Design review of the part built by this model. Coordinates are the model's own, in mm. Round coordinates to 2 decimals unless told otherwise and drop trailing zeros. Loops run counter-clockwise (first coordinate to the right, second up) from the corner with the lowest first, then second, coordinate; pieces in that order, holes last. Notation, with made-up numbers: (-15.5, 30) - (23.5, 30) arc R29 cw to (23.5, 63) - close; hole circle Ø4 at (-5.75, 14). An arc over 180 degrees is marked (long way). Return JSON: item names as keys, results as strings. Group by question number.
(1) We need section A-A, the plane x = -257.5. Write out the cut boundary in (y, z).
(2) Wall thickness on L1, parallel to Z at x = -230, y = 3.05; L2, parallel to Z at x = -247, y = 1.85; L3, parallel to X at y = 1, z = -209: over which ranges is each line inside the solid? List them lowest first. Write a range as [from, to].
(3) We need section C-C, the plane z = -112. Write out the cut boundary in (x, y), and give its area (3 significant figures).
(4) We need section B-B, the plane y = 2.65. Give the number of separate pieces and of enclosed holes in the cut face, and give its area (3 significant figures).
(5) We need section D-D, the plane x = -20. Write out the cut boundary in (y, z).
(6) Clearance check with flat-ended pins moving along their axes: pin 1 (1.8 mm diameter, centred on x = -2.5, y = 4, fed in from -Z); pin 2 (5 mm diameter, centred on x = -89.5, z = -208, fed in from -Y); pin 3 (1 mm diameter, centred on x = -182.5, y = 2, fed in from +Z); pin 4 (3 mm diameter, centred on x = -1, y = 3, fed in from +Z). State where each tip first meets the part, or that it passes through.
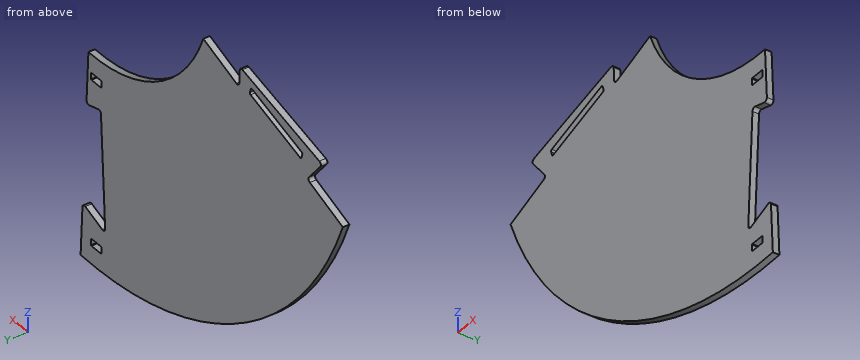
Autodesk Inventor part; units mm, degrees
ref_plane "Work Plane1" through (265.3907, 0, -86.2307) normal (0.309, 0, 0.9511) x (0.9511, 0, -0.309)
ref_plane "YZ Plane" through (0, 0, 0) normal (1, 0, 0) x (0, 1, 0)
ref_plane "XZ Plane" through (0, 0, 0) normal (0, 1, 0) x (-1, 0, 0)
sketch "Sketch1" plane through (0, 0, 0) normal (0, 1, 0) x (-1, 0, 0)
  circle A0 centre (0, 0) radius 341.36
  circle A1 centre (0, 0) radius 150.07
  dimension "d84" = 300.14
  dimension "d85" = 682.72
extrude "Extrusion3" add sketch "Sketch1" along normal blind 6 contours A0 | A1
sketch "Sketch2" plane through (0, 6, 0) normal (0, 1, 0) x (1, 0, 0)
  circle A0 centre (0, 0) radius 245.715 construction
  line L0 (245.7148, 0.3131) -> (341.6521, -0.0088)
  line L1 (-0.6289, 279.0483) -> (-0.0524, 279.0483)
  line L2 (3.25, 279.0483) -> (3.25, 212.3817)
  line L3 (0.5377, 212.3817) -> (-0.051, 212.3817)
  line L4 (-3.25, 212.3817) -> (-3.25, 279.0483)
  arc A1 (-3.25, 212.3817) -> (-1.9167, 211.0483) centre (-1.9167, 212.3817) ccw
  arc A2 (1.9167, 211.0483) -> (3.25, 212.3817) centre (1.9167, 212.3817) ccw
  arc A3 (-1.9167, 280.3817) -> (-3.25, 279.0483) centre (-1.9167, 279.0483) ccw
  arc A4 (3.25, 279.0483) -> (1.9167, 280.3817) centre (1.9167, 279.0483) ccw
  line L5 (-1.9167, 280.3817) -> (1.9167, 280.3817)
  line L6 (-1.9167, 211.0483) -> (1.9167, 211.0483)
  line L7 (0, 0) -> (0, 212.3817)
  line L8 (0, 280.3817) -> (0, 341.36)
  line L9 (0, 211.0483) -> (0, 245.715) construction
  line L10 (0, 280.3817) -> (0, 245.715) construction
  line L11 (-265.5851, 85.6325) -> (-265.4069, 86.1808)
  line L12 (-267.2511, 84.8198) -> (-266.0665, 88.4656)
  line L13 (-201.3112, 63.3947) -> (-200.1266, 67.0404)
  arc A5 (-267.2511, 84.8198) -> (-266.395, 83.1397) centre (-265.983, 84.4078) ccw
  arc A6 (-264.3864, 89.3216) -> (-266.0665, 88.4656) centre (-264.7985, 88.0535) ccw
  line L14 (-266.6588, 86.6427) -> (-233.6889, 75.9301) construction
  line L15 (-202.9913, 62.5386) -> (-266.395, 83.1397)
  line L16 (-264.3864, 89.3216) -> (-200.9827, 68.7205)
  line L17 (-200.7189, 65.2175) -> (-233.6889, 75.9301) construction
  arc A7 (-202.9913, 62.5386) -> (-201.3112, 63.3947) centre (-202.5793, 63.8067) ccw
  arc A8 (-200.1266, 67.0404) -> (-200.9827, 68.7205) centre (-201.3947, 67.4524) ccw
  line L18 (-201.8208, 66.141) -> (-202.0027, 65.5811)
  line L19 (-163.5117, -226.1245) -> (-163.9781, -225.7857)
  line L20 (-163.2536, -227.9601) -> (-166.3548, -225.7069)
  line L21 (-122.5005, -171.8683) -> (-125.6017, -169.6151)
  arc A9 (-163.2536, -227.9601) -> (-161.3912, -227.6651) centre (-162.4699, -226.8814) ccw
  arc A10 (-166.6498, -223.8445) -> (-166.3548, -225.7069) centre (-165.5711, -224.6283) ccw
  line L22 (-164.8042, -226.8335) -> (-144.4277, -198.7876) construction
  line L23 (-122.2055, -173.7307) -> (-161.3912, -227.6651)
  line L24 (-166.6498, -223.8445) -> (-127.4641, -169.9101)
  line L25 (-124.0511, -170.7417) -> (-144.4277, -198.7876) construction
  arc A11 (-122.2055, -173.7307) -> (-122.5005, -171.8683) centre (-123.2842, -172.947) ccw
  arc A12 (-125.6017, -169.6151) -> (-127.4641, -169.9101) centre (-126.3854, -170.6938) ccw
  line L26 (-125.2699, -171.5043) -> (-124.7936, -171.8503)
  line L27 (164.5293, -225.3852) -> (164.0629, -225.724)
  line L28 (166.3548, -225.7069) -> (163.2536, -227.9601)
  line L29 (125.6017, -169.6151) -> (122.5005, -171.8683)
  arc A13 (166.3548, -225.7069) -> (166.6498, -223.8445) centre (165.5711, -224.6283) ccw
  arc A14 (161.3912, -227.6651) -> (163.2536, -227.9601) centre (162.4699, -226.8814) ccw
  line L30 (164.8042, -226.8335) -> (144.4277, -198.7876) construction
  line L31 (127.4641, -169.9101) -> (166.6498, -223.8445)
  line L32 (161.3912, -227.6651) -> (122.2055, -173.7307)
  line L33 (124.0511, -170.7417) -> (144.4277, -198.7876) construction
  arc A15 (127.4641, -169.9101) -> (125.6017, -169.6151) centre (126.3854, -170.6938) ccw
  arc A16 (122.5005, -171.8683) -> (122.2055, -173.7307) centre (123.2842, -172.947) ccw
  line L34 (124.3998, -172.1365) -> (124.8761, -171.7904)
  line L35 (265.1964, 86.8288) -> (265.3745, 86.2805)
  line L36 (266.0665, 88.4656) -> (267.2511, 84.8198)
  line L37 (200.1266, 67.0404) -> (201.3112, 63.3947)
  arc A17 (266.0665, 88.4656) -> (264.3864, 89.3216) centre (264.7985, 88.0535) ccw
  arc A18 (266.395, 83.1397) -> (267.2511, 84.8198) centre (265.983, 84.4078) ccw
  line L38 (266.6588, 86.6427) -> (233.6889, 75.9301) construction
  line L39 (200.9827, 68.7205) -> (264.3864, 89.3216)
  line L40 (266.395, 83.1397) -> (202.9913, 62.5386)
  line L41 (200.7189, 65.2175) -> (233.6889, 75.9301) construction
  arc A19 (200.9827, 68.7205) -> (200.1266, 67.0404) centre (201.3947, 67.4524) ccw
  arc A20 (201.3112, 63.3947) -> (202.9913, 62.5386) centre (202.5793, 63.8067) ccw
  line L42 (202.1531, 65.1181) -> (201.9712, 65.678)
  point P0 (-201.987, 65.6295)
  point P1 (-124.8348, -171.8204)
  point P2 (124.8348, -171.8204)
  point P3 (201.987, 65.6295)
  dimension "d21" = 6.5
  dimension "d23" = 66.6667
  dimension "d24" = 2.6667
  dimension "d25" = 2.6667
  dimension "d32" = 1.3333
  dimension "d33" = 1.3333
  dimension "d41" = 90
  dimension "d42" = 3.25
  dimension "d43" = 90
  dimension "d49" = 360
  dimension "d86" = 491.43
extrude "Extrusion4" cut sketch "Sketch2" against normal through all
sketch "Sketch3" plane through (0, 6, 0) normal (0, 1, 0) x (1, 0, 0)
  arc A0 (-115.2299, -321.3234) -> (115.2355, -321.3214) centre (0, 0) ccw
  arc A1 (-77.7244, -128.3741) -> (77.7297, -128.3709) centre (0, 0) ccw
  line L0 (-122.1811, -173.696) -> (-161.3589, -227.6196)
  line L1 (-115.2299, -321.3234) -> (-77.7244, -128.3741)
  line L2 (0, 0) -> (0, -341.2918)
  line L3 (115.2355, -321.3214) -> (77.7297, -128.3709)
  line L4 (161.3912, -227.6651) -> (122.2055, -173.7307)
  dimension "d52" = 25
  dimension "d87" = 150.07
  dimension "d88" = 341.36
  dimension "d89" = 25
  dimension "d90" = 11
  dimension "d91" = 11
extrude "Extrusion5" cut sketch "Sketch3" against normal blind 10
sketch "Sketch5" plane through (0, 6, 0) normal (0, 1, 0) x (1, 0, 0)
  line L0 (3.25, 279.0483) -> (3.25, 212.3817)
  line L1 (5.5862, 197.9634) -> (-6.155, 194.8174)
  line L2 (-11.2263, 301.7146) -> (10.5847, 293.3421)
  line L3 (6.5657, 149.9554) -> (8.9394, 195.248)
  line L4 (14.2034, 295.6921) -> (16.5771, 340.9846)
  arc A0 (10.5847, 293.3421) -> (14.2034, 295.6921) centre (11.5404, 295.8316) ccw
  arc A1 (8.9394, 195.248) -> (5.5862, 197.9634) centre (6.2763, 195.3876) ccw
  arc A2 (-11.2263, 301.7146) -> (-14.8449, 299.0854) centre (-12.1819, 299.225) ccw
  line L5 (-3.25, 212.3817) -> (-3.25, 279.0483)
  line L6 (-14.8449, 299.0854) -> (-9.5081, 197.2536)
  arc A3 (-9.5081, 197.2536) -> (-6.155, 194.8174) centre (-6.8451, 197.3932) ccw
  line L7 (-1.9167, 211.0483) -> (1.9167, 211.0483)
  line L8 (1.9167, 280.3817) -> (-1.9167, 280.3817)
  arc A4 (115.2355, -321.3214) -> (-115.2299, -321.3234) centre (0, 0) ccw
  line L9 (16.5771, 340.9846) -> (16.5774, 340.9903)
  arc A5 (-190.5375, 51.9119) -> (-187.1843, 54.3482) centre (-189.8473, 54.4877) ccw
  line L10 (-186.5481, 66.4868) -> (-187.1843, 54.3482)
  arc A6 (-182.9295, 68.8368) -> (-186.5481, 66.4868) centre (-183.8851, 66.3472) ccw
  arc A7 (-275.714, 100.7144) -> (-276.8308, 104.8821) centre (-277.7864, 102.3926) ccw
  line L11 (-289.0345, 78.3041) -> (-190.5375, 51.9119)
  arc A8 (-290.4167, 82.5581) -> (-289.0345, 78.3041) centre (-288.3443, 80.8799) ccw
  line L12 (-290.4167, 82.5581) -> (-275.714, 100.7144)
  line L13 (-276.8308, 104.8821) -> (-319.1731, 121.1358)
  line L14 (-140.5872, 52.5831) -> (-182.9295, 68.8368)
  line L15 (-319.1731, 121.1358) -> (-319.1784, 121.1378)
  arc A9 (184.6611, 69.9975) -> (183.3803, 66.0556) centre (185.6168, 67.508) ccw
  line L16 (190.0006, 55.8613) -> (183.3803, 66.0556)
  arc A10 (188.4543, 51.8331) -> (190.0006, 55.8613) centre (187.7641, 54.4089) ccw
  arc A11 (282.2558, 80.581) -> (285.609, 77.8656) centre (284.9188, 80.4414) ccw
  line L17 (279.8598, 106.5409) -> (184.6611, 69.9975)
  arc A12 (283.4785, 103.9117) -> (279.8598, 106.5409) centre (280.8155, 104.0513) ccw
  line L18 (283.4785, 103.9117) -> (282.2558, 80.581)
  line L19 (285.609, 77.8656) -> (329.4183, 89.6043)
  line L20 (144.645, 40.0945) -> (188.4543, 51.8331)
  line L21 (329.4183, 89.6043) -> (329.4238, 89.6058)
  circle A13 centre (0, 0) radius 150.07
  line L22 (-140.5872, 52.5831) -> (-140.5479, 52.568)
  line L23 (144.645, 40.0945) -> (144.5122, 40.0589)
  line L24 (6.5657, 149.9554) -> (6.5621, 149.8874)
  arc A14 (-77.7244, -128.3741) -> (77.7297, -128.3709) centre (0, 0) ccw
  arc A15 (115.2355, -321.3214) -> (-115.2299, -321.3234) centre (0, 0) ccw
  line L25 (77.7297, -128.3709) -> (115.2355, -321.3214)
  line L26 (-77.7244, -128.3741) -> (-115.2299, -321.3234)
  point P0 (-77.7399, -128.3998)
  point P1 (77.7399, -128.3998)
  point P2 (-319.1475, 121.126)
  point P3 (-140.56, 52.5727)
  point P4 (6.5642, 149.9264)
  point P5 (16.5757, 340.9573)
  point P6 (329.3918, 89.5972)
  point P7 (144.6169, 40.0869)
  dimension "d63" = 2.6667
  dimension "d64" = 3
  dimension "d66" = 3
  dimension "d67" = 2.6667
  dimension "d68" = 2.6667
  dimension "d70" = 72
  dimension "d71" = 72
  dimension "d94" = 300.14
  dimension "d95" = 682.72
sketch "Sketch6" plane through (0, 6, 0) normal (0, 1, 0) x (1, 0, 0)
  line L0 (188.7727, -264.2184) -> (198.4809, -257.165)
  line L1 (194.6603, -251.9064) -> (184.9521, -258.9598)
  line L2 (161.3912, -227.6651) -> (122.2055, -173.7307)
  line L3 (166.3548, -225.7069) -> (163.2536, -227.9601)
  arc A0 (195.5915, -252.0539) -> (194.6603, -251.9064) centre (195.0522, -252.4457) ccw
  arc A1 (198.4809, -257.165) -> (198.6284, -256.2338) centre (198.0891, -256.6256) ccw
  arc A2 (187.8415, -264.0709) -> (188.7727, -264.2184) centre (188.3809, -263.6791) ccw
  arc A3 (184.9521, -258.9598) -> (184.8046, -259.891) centre (185.344, -259.4991) ccw
  line L4 (184.8046, -259.891) -> (187.8415, -264.0709)
  line L5 (198.6284, -256.2338) -> (195.5915, -252.0539)
  line L6 (122.2055, -173.7307) -> (161.3912, -227.6651)
  line L7 (141.7983, -200.6979) -> (147.057, -196.8773)
  line L8 (166.6498, -223.8445) -> (127.4641, -169.9101)
  line L9 (95.9027, -136.3937) -> (105.6109, -129.3403)
  line L10 (109.4315, -134.5989) -> (99.7233, -141.6523)
  arc A4 (109.4315, -134.5989) -> (109.579, -133.6677) centre (109.0396, -134.0596) ccw
  arc A5 (106.5421, -129.4878) -> (105.6109, -129.3403) centre (106.0027, -129.8796) ccw
  arc A6 (95.9027, -136.3937) -> (95.7552, -137.3249) centre (96.2945, -136.9331) ccw
  arc A7 (98.7921, -141.5048) -> (99.7233, -141.6523) centre (99.3314, -141.113) ccw
  line L11 (98.7921, -141.5048) -> (95.7552, -137.3249)
  line L12 (106.5421, -129.4878) -> (109.579, -133.6677)
  point P0 (0, 0)
  dimension "d104" = 6.5
  dimension "d105" = 12
  dimension "d108" = 1.3333
  dimension "d109" = 1.3333
  dimension "d110" = 1.3333
  dimension "d111" = 1.3333
  dimension "d112" = 0
  dimension "d149" = 145
  dimension "d150" = 90
  dimension "d151" = 90
  dimension "d152" = 90
  dimension "d153" = 90
extrude "Extrusion7" cut sketch "Sketch6" against normal through all
ref_plane "Work Plane1" through (265.3907, 0, -86.2307) normal (0.309, 0, 0.9511) x (0.9511, 0, -0.309)
pattern_circular "Circular Pattern2" count 2 over 72 about axis through (0, -10, 0) along (0, 1, 0) of "Extrusion7"
pattern_circular "Circular Pattern3" count 2 over 144 about axis through (0, -10, 0) along (0, 1, 0) of "Extrusion7"
mirror "Mirror3" about plane through (0, 0, 0) normal (1, 0, 0) of "Extrusion7"
pattern_circular "Circular Pattern4" count 2 over 144 about axis through (0, -10, 0) along (0, -1, 0) of "Extrusion7"
extrude "Extrusion10" cut sketch "Sketch5" against normal through all contours L1 A3 L6 A2 L2 A0 L4 A4 L19 A11 L18 A12 L17 A9 L16 A10 L20 L23 A13 L24 L3 A1 | A13 | L23 L20 A10 L16 A9 L17 A12 L18 A11 L19 A4 L25 A13 | A13 L26 A4 L13 A7 L12 A8 L11 A5 L10 A6 L14 L22
equation "\"BendRadius\" = Thickness"
equation "\"BendReliefWidth\" = Thickness"
equation "\"BendReliefDepth\" = 0.5 * Thickness"
equation "\"CornerReliefSize\" = 4 * Thickness"
equation "\"MinimumRemnant\" = 2 * Thickness"
equation "\"TransitionRadius\" = BendRadius"
equation "\"JacobiRadiusSize\" = BendRadius"
equation "\"GapSize\" = Thickness"
properties part number "Ring D2" material "Wood (Maple)"
Solutions:
{
 "1": {"outline": "(0, -224.1) - (6, -224.1) - (6, -87.08) - (0, -87.08) - close; (0, -80.25) - (6, -80.25) - (6, -69.85) - (0, -69.85) - close"},
 "2": {"L1": "[-252.24, -78.15], [-71.31, -62.49]", "L2": "[-235.62, -83.67], [-76.84, -67.04]", "L3": "[-269.9, -10.12]"},
 "3": {"outline": "(-295.37, 0) - (-99.88, 0) - (-99.88, 6) - (-295.37, 6) - close", "area": "1,170 mm^2"},
 "4": {"separate pieces": "1", "enclosed holes": "3", "area": "58,400 mm^2"},
 "5": {"outline": "(0, -340.77) - (6, -340.77) - (6, -148.73) - (0, -148.73) - close"},
 "6": {"pin 1": "z = -341.36", "pin 2": "y = 0", "pin 3": "z = -68.48", "pin 4": "z = -150.05"}
}
